Geometry: final body of the model. Coordinates: model frame, mm. Face numbers are marked on the shaded views. A direction names the side the tool comes from. Give positions to 0.01 mm unless a question says otherwise; leave off trailing zeros. Loops run counter-clockwise (first coordinate to the right, second up) from the corner with the lowest first, then second, coordinate; pieces in that order, holes last.
1. Section A-A, the plane z = 0. Output: boundary loops of the cut face in (x, y).
2. First-contact query: P1, Ø5.5, axis at y = -10, z = 0, coming from the -X side; P2, Ø2, axis at y = 0, z = 10, coming from the -X side; P3, Ø2, axis at x = 1.5, y = -5, coming from the -Z side. Flat tips, straight axial feed; report the tip coordinate or a pass-through.
3. Material intervals for line 1 along Z through (x, y) = (3.05, 0); line 2 along Y through (x, z) = (4.5, 0.25); line 3 along X through (y, z) = (7, -5.25), sorted ascending.
4. Access query for the marked faces 1 and 2. Directions: +Z, -Z, +X, -X, +Y, -Y. A direction counts if a zero-diameter tool reaches every point of the face in a straight line with its end or side. Return the directions, or none.
5. Draft query along Y for the marked faces 3, 4 and 5. Return one class per face: +Y half, -Y half, draft (parallel to the pull), parting line (faces both ways), or undercut.
6. Section B-B, the plane y = 10. Output: boundary loops of the cut face in (x, z), then the cut area to 3 significant figures.
7. Section C-C, the plane x = 4.5. Output: boundary loops of the cut face in (y, z), then the cut area to 3 significant figures.
Autodesk Inventor part; units mm, degrees
ref_plane "YZ Plane" through (0, 0, 0) normal (1, 0, 0) x (0, 1, 0)
ref_plane "XZ Plane" through (0, 0, 0) normal (0, 1, 0) x (-1, 0, 0)
ref_plane "XY Plane" through (0, 0, 0) normal (0, 0, 1) x (1, 0, 0)
sketch "Sketch_1" plane through (0, 0, 0) normal (0, 0, 1) x (1, 0, 0)
  line L0 (16, 0) -> (0, 0)
  line L1 (0, 4) -> (16, 4)
  line L2 (16, 4) -> (16, 6)
  line L3 (16, 6) -> (5, 6)
  line L4 (5, 6) -> (5, 14)
  line L5 (5, 14) -> (0, 14)
  line L6 (0, 14) -> (0, 4)
revolve "Revolution1" add sketch "Sketch_1" angle 360 about axis through (16, 0, 0) along (1, 0, 0)
sketch "Sketch_3" plane through (0, 0, 0) normal (0, -0.7071, 0.7071) x (1, 0, 0)
  line L0 (10, 3.5) -> (10, 6)
  line L1 (10, 6) -> (11.5, 6)
  line L2 (11.5, 6) -> (11.2295, 5.7295)
  line L3 (11.2295, 5.7295) -> (11.2295, 3.5)
  line L4 (11.2295, 3.5) -> (10, 3.5)
  line L5 (10, 3.5) -> (10, 6)
revolve "Revolution2" cut sketch "Sketch_3" angle 360 about axis through (10, 2.4749, 2.4749) along (0, -0.7071, -0.7071)
thread "Thread1"
sketch "Sketch3" plane through (5, 0, 0) normal (1, 0, 0) x (0, 0, -1)
  point P0 (0, 10)
hole "Hole1" at (5, 10, 0) direction (-1, 0, 0) diameter 3.5 depth 5
sketch "Sketch4" plane through (5, 0, 0) normal (1, 0, 0) x (0, 0, -1)
  point P0 (0, -10)
hole "Hole2" at (5, -10, 0) direction (-1, 0, 0) diameter 3.5 depth 5
sketch "Sketch5" plane through (5, 0, 0) normal (1, 0, 0) x (0, 0, -1)
  point P0 (-10, 0)
hole "Hole3" at (5, 0, 10) direction (-1, 0, 0) diameter 3.5 depth 5
sketch "Sketch6" plane through (5, 0, 0) normal (1, 0, 0) x (0, 0, -1)
  point P0 (10, 0)
hole "Hole4" at (5, 0, -10) direction (-1, 0, 0) diameter 3.5 depth 5
sketch "Sketch_2" plane through (0, 0, 0) normal (0, -0.7071, -0.7071) x (1, 0, 0)
  line L0 (10, 3.5) -> (10, 6)
  line L1 (10, 6) -> (11.5, 6)
  line L2 (11.5, 6) -> (11.2295, 5.7295)
  line L3 (11.2295, 5.7295) -> (11.2295, 3.5)
  line L4 (11.2295, 3.5) -> (10, 3.5)
  line L5 (10, 3.5) -> (10, 6)
revolve "Revolution3" cut sketch "Sketch_2" angle 360 about axis through (10, -2.4749, 2.4749) along (0, 0.7071, -0.7071)
thread "Thread2"
properties part number "STHRB8_b"
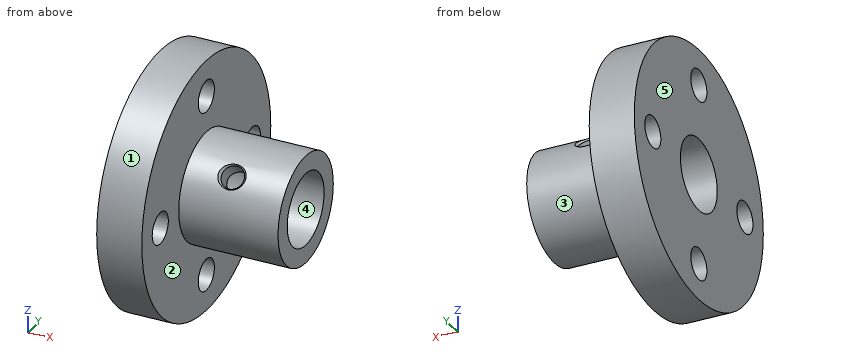
Answers below:
1. outline: (0, -14) - (5, -14) - (5, -11.75) - (0, -11.75) - close; (0, -8.25) - (5, -8.25) - (5, -6) - (16, -6) - (16, -4) - (0, -4) - close; (0, 4) - (16, 4) - (16, 6) - (5, 6) - (5, 8.25) - (0, 8.25) - close; (0, 11.75) - (5, 11.75) - (5, 14) - (0, 14) - close
2. P1: stops at x = 0
2. P2: passes through
2. P3: stops at z = -13.42
3. line 1: z = -14 to -11.75, -8.25 to -4, 4 to 8.25, 11.75 to 14
3. line 2: y = -14 to -11.73, -8.27 to -3.99, 3.99 to 8.27, 11.73 to 14
3. line 3: x = 0 to 5
4. face 1: +X, -X
4. face 2: +X
5. face 3: parting line
5. face 4: undercut
5. face 5: draft
6. outline: (0, -9.8) - (5, -9.8) - (5, -1.75) - (0, -1.75) - close; (0, 1.75) - (5, 1.75) - (5, 9.8) - (0, 9.8) - close
6. area: 80.5 mm2
7. outline: circle Ø28 at (0, 0); hole circle Ø3.5 at (-10, 0); hole circle Ø8 at (0, 0); hole circle Ø3.5 at (0, -10); hole circle Ø3.5 at (0, 10); hole circle Ø3.5 at (10, 0)
7. area: 527 mm2
